Here's how the part is built. I have some questions about the finished solid (model axes, mm). Face numbers are marked on the shaded views. A direction names the side the tool comes from. Round coordinates to 2 decimals unless told otherwise and drop trailing zeros. Write each loop counter-clockwise with the first axis right and the second up, starting at its lowest first coordinate (ties: lowest second). Pieces come first, ordered by that corner, then holes. Notation, with made-up numbers: (21.5, -39.75) -> (56.5, -39.75) arc R27 ccw to (56.5, -14.75) -> close; hole circle Ø4 at (53.25, 79.25). An arc over 180 degrees is marked (long way). Put each result on its own line as item: value. Start each with the question number.
1. Suppose I cut it at A-A (x = 10.1). Please give me the cut outline in (y, z), then the cut area to 3 significant figures.
2. Suppose I cut it at B-B (y = 12). Please give me the cut outline in (x, z), then the cut area to 3 significant figures.
3. Which directions (+Z, -Z, +X, -X, +Y, -Y) give clear straight access to the entire face, cutting with the end or side of a thin tool? Please do the marked faces 4, 5, 6, 7 and 8.
4. Suppose I cut it at C-C (y = 15.75). Please give me the cut outline in (x, z).
5. I need wall thicknesses on probe 1 along X at (y, z) = (17, 0.65); probe 2 along Y at (x, z) = (10.1, 3.05); probe 3 along Y at (x, z) = (3.5, 0.55). Which ranges of each line are inside material? Lowest first, please. Write a range as from..to.
6. For pin 1 (3.5 mm diameter, centred on x = 7.43, y = 16.54, fed in from +Z); pin 2 (3 mm diameter, centred on x = 15, y = 10.5, fed in from +Z); pin 3 (3 mm diameter, centred on x = 4, z = 4.5, fed in from +Y); pin 4 (1 mm diameter, centred on y = 6, z = 3.5, fed in from -X), each with a flat end and sliding along its axis, tell me the tip position at first contact or that it passes through.
7. We'd pull the mould along Y, two halves only. Please class the marked faces 1, 2 and 3: +Y half, -Y half, draft (parallel to the pull), parting line (faces both ways), or undercut.
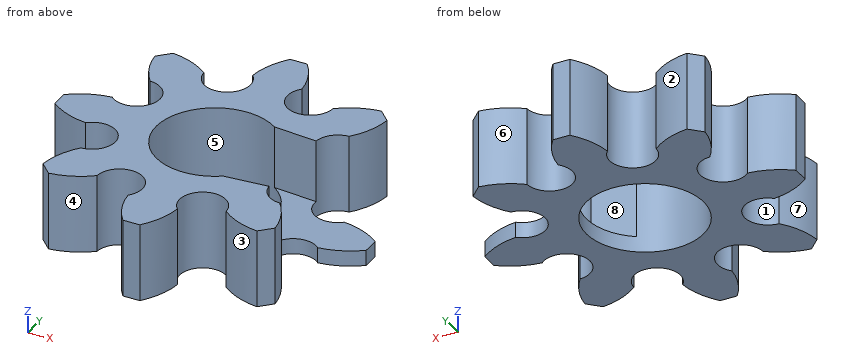
```python
from build123d import *

# Parameters (mm, degrees)
SKETCH1_R           = 3.75
BOSS_EXTRUDE1_DEPTH = 5
CUT_EXTRUDE1_DEPTH  = 4


with BuildPart() as part:
    # Sketch1 → Boss-Extrude1 (new body)
    with BuildSketch(Plane.XY):
        with BuildLine():
            Line((9.558996201, 20.085353851), (10.641002655, 20.085353851))
            ThreePointArc((10.641002655, 20.085353851), (11.348612191, 18.888750883), (11.682733536, 17.539331436))
            ThreePointArc((11.682733536, 17.539331436), (12.203470274, 15.178225243), (14.241240442, 16.479563766))
            ThreePointArc((14.241240442, 16.479563766), (15.432774832, 17.194885225), (16.778165126, 17.543258511))
            Line((16.778165126, 17.543258511), (17.543259228, 16.77816441))
            ThreePointArc((17.543259228, 16.77816441), (17.197488656, 15.431682836), (16.479564483, 14.241239725))
            ThreePointArc((16.479564483, 14.241239725), (15.178226761, 12.203469046), (17.539333159, 11.682733236))
            ThreePointArc((17.539333159, 11.682733236), (18.887683861, 11.345999843), (20.085355575, 10.641002355))
            Line((20.085355575, 10.641002355), (20.085355575, 9.558995901))
            ThreePointArc((20.085355575, 9.558995901), (18.888752607, 8.851386365), (17.539333159, 8.51726502))
            ThreePointArc((17.539333159, 8.51726502), (15.178226966, 7.996528282), (16.479565489, 5.958758114))
            ThreePointArc((16.479565489, 5.958758114), (17.194886948, 4.767223724), (17.543260234, 3.42183343))
            Line((17.543260234, 3.42183343), (16.778166133, 2.656739328))
            ThreePointArc((16.778166133, 2.656739328), (15.431684559, 3.0025099), (14.241241448, 3.720434073))
            ThreePointArc((14.241241448, 3.720434073), (12.203470769, 5.021771795), (11.682734959, 2.660665397))
            ThreePointArc((11.682734959, 2.660665397), (11.346001566, 1.312314695), (10.641004079, 0.114642981))
            Line((10.641004079, 0.114642981), (9.558997624, 0.114642981))
            ThreePointArc((9.558997624, 0.114642981), (8.851388089, 1.311245949), (8.517266743, 2.660665397))
            ThreePointArc((8.517266743, 2.660665397), (7.996530005, 5.02177159), (5.958759838, 3.720433067))
            ThreePointArc((5.958759838, 3.720433067), (4.767225448, 3.005111608), (3.421835153, 2.656738322))
            Line((3.421835153, 2.656738322), (2.656741052, 3.421832423))
            ThreePointArc((2.656741052, 3.421832423), (3.002511624, 4.768313997), (3.720435797, 5.958757108))
            ThreePointArc((3.720435797, 5.958757108), (5.021773518, 7.996527787), (2.66066712, 8.517263597))
            ThreePointArc((2.66066712, 8.517263597), (1.312316418, 8.85399699), (0.114644705, 9.558994477))
            Line((0.114644705, 9.558994477), (0.114644705, 10.641000932))
            ThreePointArc((0.114644705, 10.641000932), (1.311247673, 11.348610467), (2.66066712, 11.682731813))
            ThreePointArc((2.66066712, 11.682731813), (5.021773313, 12.203468551), (3.72043479, 14.241238718))
            ThreePointArc((3.72043479, 14.241238718), (3.005113331, 15.432773108), (2.656740045, 16.778163403))
            Line((2.656740045, 16.778163403), (3.421834146, 17.543257504))
            ThreePointArc((3.421834146, 17.543257504), (4.76831572, 17.197486932), (5.958758831, 16.479562759))
            ThreePointArc((5.958758831, 16.479562759), (7.99652951, 15.178225038), (8.51726532, 17.539331436))
            ThreePointArc((8.51726532, 17.539331436), (8.853998713, 18.887682137), (9.558996201, 20.085353851))
        make_face()
        with Locations((10.099999428, 10.099999428)):
            Circle(SKETCH1_R, mode=Mode.SUBTRACT)
    extrude(amount=BOSS_EXTRUDE1_DEPTH)

    # Sketch2 → Cut-Extrude1 (cut)
    with BuildSketch(Plane.XY.offset(5)):
        Polygon((12.190990541, 13.162654627), (12.274208264, 7.044624502), (15.074227333, 7.289583683), (15.112805831, 7.292958716), (23.65344112, 8.040134707), (23.65344112, 12.159866086), (15.074227333, 12.910415649), align=None)
    extrude(amount=-CUT_EXTRUDE1_DEPTH, mode=Mode.SUBTRACT)


solid = part.part
```
Verdict:
1. outline: (0.11, 0) -> (6.35, 0) -> (6.35, 5) -> (0.11, 5) -> close; (13.85, 0) -> (20.09, 0) -> (20.09, 5) -> (13.85, 5) -> close
1. area: 62.4 mm^2
2. outline: (4.92, 0) -> (6.87, 0) -> (6.87, 5) -> (4.92, 5) -> close; (13.33, 0) -> (15.28, 0) -> (15.28, 1) -> (13.33, 1) -> close
2. area: 11.7 mm^2
3. face 4: +Z, -Z, -Y
3. face 5: +Z, -Z
3. face 6: +Z, -Z, +Y
3. face 7: +Z, -Z, -X
3. face 8: +Z
4. outline: (2.88, 0) -> (6.19, 0) -> (6.19, 5) -> (2.88, 5) -> close; (8.68, 0) -> (11.52, 0) -> (11.52, 5) -> (8.68, 5) -> close; (14.01, 0) -> (17.32, 0) -> (17.32, 5) -> (14.01, 5) -> close
5. probe 1: x = 2.88..5.18, 8.83..11.37, 15.02..17.32
5. probe 2: y = 0.11..6.35, 13.85..20.09
5. probe 3: y = 2.67..5.67, 8.9..11.3, 14.53..17.53
6. pin 1: stops at z = 5
6. pin 2: stops at z = 1
6. pin 3: stops at y = 17.54
6. pin 4: stops at x = 3.39
7. face 1: undercut
7. face 2: +Y half
7. face 3: -Y half
